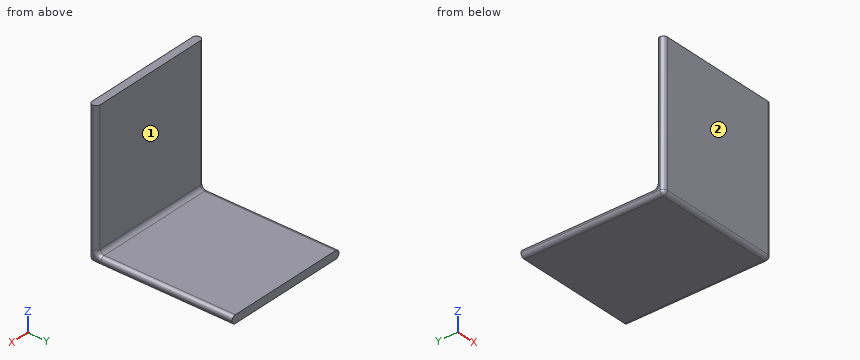
from build123d import *

# Parameters (mm, degrees)
F0_W     = 10
F0_H     = 170
F0_H_2   = 10
F0_W_2   = 170
F1_DEPTH = 160
F2_R     = 4.99999


# Not quite as in the source:
# - a fillet or chamfer is up to 0.001 mm smaller than in the source, because OpenCascade refuses the exact size


with BuildPart() as f1:
    # F0 (on Right) → F1 (new body)
    with BuildSketch(Plane.YZ):
        with Locations((-40.9939204156, 85)):
            Rectangle(F0_W, F0_H)
        with Locations((-40.9939204156, -5)):
            Rectangle(F0_W, F0_H_2)
        with Locations((49.0060795844, -5)):
            Rectangle(F0_W_2, F0_H_2)
    extrude(amount=-F1_DEPTH)

    # F2 (radius 5 in the source; OpenCascade refuses exactly that, so slightly less here)
    f2_edges = [f1.edges().sort_by_distance(p)[0] for p in [
        (0, 49.00608, 0),
        (0, 44.00608, -10),
        (-160, 49.00608, 0),
        (-160, 44.00608, -10),
        (-80, -35.99392, 0),
        (-160, -35.99392, 85),
        (-160, -45.99392, 80),
        (0, -35.99392, 85),
        (0, -45.99392, 80),
        (-80, -45.99392, -10),
    ]]
    fillet(f2_edges, radius=F2_R)


solid = f1.part
For this review, take the finished solid that the model builds, in its own axes (mm). Face numbers are marked on the shaded views. A direction names the side the tool comes from. Give positions to 0.01 mm unless a question says otherwise; leave off trailing zeros. Put each result on its own line as item: value. Start each with the question number.
(1) Machinability: for the marked faces 1 and 2, which of the approach directions +Z, -Z, +X, -X, +Y, -Y give a long, thin tool a straight path to every point of the face, cutting with its end or side? Answer none if there is none.
(2) For pin 1 (10 mm diameter, centred on x = -123.5, z = 137.5, fed in from +Y); pin 2 (4 mm diameter, centred on x = -34, y = 10, fed in from +Z), all flat-tipped, find the tip position at first contact; note any pin that passes through.
(3) Wall thickness on L1, parallel to Y at x = -133.5, z = 51.5; L2, parallel to Z at x = -120, y = 55: over which ranges is each line inside the solid? List them lowest first.
Result:
1. face 1: +Z, +X, -X, +Y
1. face 2: +Z, -Z, +X, -X, -Y
2. pin 1: stops at y = -35.99
2. pin 2: stops at z = 0
3. L1: y = -45.99 to -35.99
3. L2: z = -10 to 0
